The listing builds one solid part. Answer for the finished solid, in the listing's coordinates (mm). A direction names the side the tool comes from. Give positions to 0.01 mm unless a question says otherwise; leave off trailing zeros. Order: outer loops, then holes, each group sorted by start corner. A loop starts at its lowest first (then second) coordinate and runs counter-clockwise, first axis right, second up.
```python
from build123d import *

# Parameters (mm, degrees)
PAD_DEPTH   = 11
FILLET_R    = 1
FILLET001_R = 1


with BuildPart() as part:
    # Sketch → Pad (new body)
    with BuildSketch(Plane.XZ):
        with BuildLine():
            Line((0, 0), (0, 18.468932))
            Line((0, 18.468932), (-9, 18.468932))
            ThreePointArc((-9, 18.468932), (-14.55271, 18.309956), (-19.383095, 15.566739))
            Line((-17.314404, 13.868706), (-19.383095, 15.566739))
            ThreePointArc((-18.083851, 1.368706), (-2.623704, 6.690727), (-17.314404, 13.868706))
            Line((-18.083851, 1.368706), (-20.396363, 0))
            ThreePointArc((-20.396363, 0), (-15.265575, -3.616554), (-9, -4))
            Line((-9, -4), (0, -4))
            Line((0, 0), (0, -4))
        make_face()
    extrude(amount=PAD_DEPTH)

    # Fillet
    fillet_edges = [part.edges().sort_by_distance(p)[0] for p in [
        (-18.083851, -5.5, 1.368706),
        (-20.396363, -5.5, 0),
        (-19.240107, 0, 0.684353),
        (-19.240107, -11, 0.684353),
    ]]
    fillet(fillet_edges, radius=FILLET_R)

    # Fillet001
    fillet001_edges = [part.edges().sort_by_distance(p)[0] for p in [
        (-17.314404, -5.5, 13.868706),
        (-19.383095, -5.5, 15.566739),
        (-18.348749, 0, 14.717723),
        (-18.348749, -11, 14.717723),
    ]]
    fillet(fillet001_edges, radius=FILLET001_R)

    # Mirrored: part across YZ


with BuildPart() as part_1:
    add(part.part)
    add(part.part.mirror(Plane.YZ))


solid = part_1.part
```
1) Find section A-A (x = -13.5). Write down the section's boundary in (y, z), then the cut area to 3 significant figures.
Geometry says:
outline: (-11, -4.08) - (0, -4.08) - (0, -1.38) - (-11, -1.38) - close; (-11, 15.85) - (0, 15.85) - (0, 18.55) - (-11, 18.55) - close
area: 59.5 mm2
2) For a pull along X with two mould halves and no side action, classify faces 1 (the cylindrical face through (17.94, -10.81, 14.92)), 2 (the cylindrical face through (-18.826, -5.577, 15.587)), 3 (the cylindrical face through (-2.646, -5.423, 6.399)), 4 (the flat face through (0, -11, 6)) as +X half, -X half, draft (parallel to the pull), parting line (faces both ways), or undercut.
Geometry says:
face 1: +X half
face 2: -X half
face 3: undercut
face 4: draft
3) Given P1, Ø3.5, axis at x = 1.5, y = -4.5, coming from the -Z side; P2, Ø5.5, axis at x = -3, y = -7, coming from the +Z side; P3, Ø4, axis at y = -7, z = 4.5, coming from the +X side, each flat-ended and moving along its own axis, determine where each tip first touches the part or whether it passes through.
Geometry says:
P1: stops at z = -4
P2: stops at z = 18.47
P3: stops at x = 3.98
4) A tool of negligible diameter and unlimited length cuts with its end or side. For faces 5 (the cylindrical face through (18.84, -10.81, 0.44)), 6 (the cylindrical face through (-17.33, -5.58, 14.16)), 7 (the cylindrical face through (17.927, -0.175, 14.935)), 8 (the cylindrical face through (-17.927, -0.175, 14.935)), from which of +Z, -Z, +X, -X, +Y, -Y can it reach the whole face along a straight path? Write none if from no direction.
Geometry says:
face 5: +X, -Y
face 6: +Y, -Y
face 7: +X, +Y
face 8: -X, +Y
5) Straight lines are drawn through the part: probe 1 along Z at (x, y) = (5, -5.5); probe 2 along Z at (x, y) = (-10, -2); probe 3 along X at (y, z) = (-7, 14.75). For each, find the intervals that lie inside material, in ascending order.
Geometry says:
probe 1: z = -4 to 1.18, 13.29 to 18.47
probe 2: z = -4.17 to -1.49, 15.96 to 18.64
probe 3: x = -18.39 to -16.13, -6.78 to 6.78, 16.13 to 18.39
6) Find section B-B (y = -8). Write down the section's boundary in (x, z).
Geometry says:
outline: (-19.54, -0.95) arc R11.5 ccw to (-9, -4) - (9, -4) arc R11.5 ccw to (19.54, -0.95) arc R1 ccw to (19.34, 0.62) - (18.76, 0.97) arc R1 ccw to (17.56, 0.83) arc R8.85 cw (long way) to (16.71, 14.35) arc R1 ccw to (17.94, 14.38) - (18.46, 14.81) arc R1 ccw to (18.43, 16.38) arc R11.5 ccw to (9, 18.47) - (-9, 18.47) arc R11.5 ccw to (-18.43, 16.38) arc R1 ccw to (-18.46, 14.81) - (-17.94, 14.38) arc R1 ccw to (-16.71, 14.35) arc R8.85 cw (long way) to (-17.56, 0.83) arc R1 ccw to (-18.76, 0.97) - (-19.34, 0.62) arc R1 ccw to start
7) Find section D-D (z = 8). Write down the section's boundary in (x, y), then the cut area to 3 significant figures.
Geometry says:
outline: (-2.64, -11) - (2.64, -11) - (2.64, 0) - (-2.64, 0) - close
area: 58.1 mm2
8) Find section C-C (x = -6.5). Write down the section's boundary in (y, z).
Geometry says:
outline: (-11, -4) - (0, -4) - (0, -0.1) - (-11, -0.1) - close; (-11, 14.57) - (0, 14.57) - (0, 18.47) - (-11, 18.47) - close
